Geometry check sheet. Reference: the model listing, model coordinates, mm. A direction names the side the tool comes from. Round coordinates to 2 decimals unless told otherwise and drop trailing zeros. Write each loop counter-clockwise with the first axis right and the second up, starting at its lowest first coordinate (ties: lowest second). Pieces come first, ordered by that corner, then holes. Notation, with made-up numbers: M 37,-39 L 72,-39 A25 cw 72,-18 Z; hole C 3.25,71.25 d9. An arc over 180 degrees is marked long. Answer as CSV lines item,"result". Start each with the question number.
```python
from build123d import *

# Parameters (mm, degrees)
SKETCH1_W                = 150
SKETCH1_H                = 1500
SKETCH1_W_2              = 110
SKETCH1_H_2              = 1460
BOSS_EXTRUDE1_DEPTH      = 20
SKETCH2_W                = 20
SKETCH2_H                = 20
BOSS_EXTRUDE2_DEPTH      = 640
SKETCH3_W                = 150
SKETCH3_H                = 1500
SKETCH3_W_2              = 110
SKETCH3_H_2              = 1460
BOSS_EXTRUDE3_DEPTH      = 20
SKETCH4_W                = 20
SKETCH4_H                = 20
BOSS_EXTRUDE4_DEPTH      = 660
SKETCH5_W                = 20
SKETCH5_H                = 20
BOSS_EXTRUDE5_DEPTH      = 600
BOSS_EXTRUDE5_DEPTH_BACK = 130
SKETCH6_W                = 140
SKETCH6_H                = 20
BOSS_EXTRUDE6_DEPTH      = 20
SKETCH7_W                = 20
SKETCH7_H                = 20
BOSS_EXTRUDE7_DEPTH      = 300
BOSS_EXTRUDE8_START      = -1480
SKETCH8_W                = 20
SKETCH8_H                = 20
BOSS_EXTRUDE8_DEPTH      = 1460


with BuildPart() as part:
    # Sketch1 → Boss-Extrude1 (new body)
    with BuildSketch(Plane(origin=(0, 0, 0), x_dir=(1, 0, 0), z_dir=(0, 1, 0))):
        with Locations((675, 0)):
            Rectangle(SKETCH1_W, SKETCH1_H)
        with Locations((675, 0)):
            Rectangle(SKETCH1_W_2, SKETCH1_H_2, mode=Mode.SUBTRACT)
    extrude(amount=BOSS_EXTRUDE1_DEPTH)

    # Sketch2 → Boss-Extrude2 (add)
    with BuildSketch(Plane(origin=(0, 20, 0), x_dir=(1, 0, 0), z_dir=(0, 1, 0))):
        with Locations((610, 740)):
            Rectangle(SKETCH2_W, SKETCH2_H)
        with Locations((740, 740)):
            Rectangle(SKETCH2_W, SKETCH2_H)
        with Locations((610, -740)):
            Rectangle(SKETCH2_W, SKETCH2_H)
        with Locations((740, -740)):
            Rectangle(SKETCH2_W, SKETCH2_H)
    extrude(amount=BOSS_EXTRUDE2_DEPTH)

    # Sketch3 → Boss-Extrude3 (add)
    with BuildSketch(Plane(origin=(0, 660, 0), x_dir=(1, 0, 0), z_dir=(0, 1, 0))):
        with Locations((675, 0)):
            Rectangle(SKETCH3_W, SKETCH3_H)
        with Locations((675, 0)):
            Rectangle(SKETCH3_W_2, SKETCH3_H_2, mode=Mode.SUBTRACT)
    extrude(amount=BOSS_EXTRUDE3_DEPTH)

    # Sketch4 → Boss-Extrude4 (add)
    with BuildSketch(Plane.XZ):
        with Locations((740, 0)):
            Rectangle(SKETCH4_W, SKETCH4_H)
        with Locations((610, 0)):
            Rectangle(SKETCH4_W, SKETCH4_H)
    extrude(amount=-BOSS_EXTRUDE4_DEPTH)

    # Sketch5 → Boss-Extrude5 (add, two sides)
    with BuildSketch(Plane.ZY.offset(-600)) as boss_extrude5_sk:
        with Locations((-740, 410)):
            Rectangle(SKETCH5_W, SKETCH5_H)
        with Locations((-740, 670)):
            Rectangle(SKETCH5_W, SKETCH5_H)
        with Locations((740, 410)):
            Rectangle(SKETCH5_W, SKETCH5_H)
        with Locations((740, 670)):
            Rectangle(SKETCH5_W, SKETCH5_H)
        with Locations((0, 670)):
            Rectangle(SKETCH5_W, SKETCH5_H)
    extrude(amount=BOSS_EXTRUDE5_DEPTH)
    extrude(boss_extrude5_sk.sketch, amount=-BOSS_EXTRUDE5_DEPTH_BACK)

    # Sketch6 → Boss-Extrude6 (add)
    with BuildSketch(Plane.XZ):
        with Locations((820, 740)):
            Rectangle(SKETCH6_W, SKETCH6_H)
        with Locations((820, 0)):
            Rectangle(SKETCH6_W, SKETCH6_H)
        with Locations((820, -740)):
            Rectangle(SKETCH6_W, SKETCH6_H)
    extrude(amount=-BOSS_EXTRUDE6_DEPTH)

    # Sketch7 → Boss-Extrude7 (add)
    with BuildSketch(Plane.XZ):
        with Locations((610, 740)):
            Rectangle(SKETCH7_W, SKETCH7_H)
        with Locations((880, 740)):
            Rectangle(SKETCH7_W, SKETCH7_H)
        with Locations((610, 0)):
            Rectangle(SKETCH7_W, SKETCH7_H)
        with Locations((610, -740)):
            Rectangle(SKETCH7_W, SKETCH7_H)
        with Locations((880, -740)):
            Rectangle(SKETCH7_W, SKETCH7_H)
        with Locations((880, 0)):
            Rectangle(SKETCH7_W, SKETCH7_H)
    extrude(amount=BOSS_EXTRUDE7_DEPTH)

    # Sketch8 → Boss-Extrude8 (add)
    with BuildSketch(Plane.XY.offset(750).offset(BOSS_EXTRUDE8_START)):
        with Locations((610, -290)):
            Rectangle(SKETCH8_W, SKETCH8_H)
        with Locations((880, -290)):
            Rectangle(SKETCH8_W, SKETCH8_H)
    extrude(amount=BOSS_EXTRUDE8_DEPTH)

    # Mirror1: part across plane


with BuildPart() as part_1:
    add(part.part)
    add(part.part.mirror(Plane(origin=(0, 0, 0), x_dir=(0, 0, 1), z_dir=(1, 0, 0))))


solid = part_1.part
```
1) Section check C-C, the plane z = -349.5. Give the number of separate pieces and of enclosed holes in the cut face, plus the area to 3 significant figures.
2) Go/stop test with flat-tipped pins: pin 1 (16 mm diameter, centred on y = 13.5, z = 478.5, fed in from -X); pin 2 (16 mm diameter, centred on y = 523.5, z = -742, fed in from +X); pin 3 (6 mm diameter, centred on x = 152.5, z = -736.5, fed in from -Y). Record where each tip stops, or that it passes through.
3) Mould release check, pull along Y, two halves, no side actions. Record for faces 1 (the flat face through (4, 410, -730)), 2 (the flat face through (-4, 680, -4)), 3 (the flat face through (872, -86, -730)): released by +Y, released by -Y, zero draft, split by the parting line, or undercut.
4) Scan line: line 1 (Z direction, x = 669, y = 414). Record every from-to range of solid material in increasing order. Write a range as from..to.
5) Section check A-A, the plane x = -193. Record the cut outline in (y, z).
6) Section check B-B, the plane x = -677. Record the cut outline in (y, z).
7) Access from +Z, -Z, +X, -X, +Y, -Y to the whole of each face (thin tool, end or side, straight path). Record for faces 4 (the flat face through (4, 410, 730)), 5 (the flat face through (-750, 495, 4)), 6 (the flat face through (754, 0, 4)).
Results:
1,separate pieces,"12"
1,enclosed holes,"0"
1,area,"4,800 mm^2"
2,pin 1,"stops at x = -750"
2,pin 2,"stops at x = 750"
2,pin 3,"stops at y = 400"
3,face 1,"undercut"
3,face 2,"released by +Y"
3,face 3,"zero draft"
4,line 1,"z = -750..-730, 730..750"
5,outline,"M 400,-750 L 420,-750 L 420,-730 L 400,-730 Z; M 400,730 L 420,730 L 420,750 L 400,750 Z; M 660,-750 L 680,-750 L 680,-730 L 660,-730 Z; M 660,-10 L 680,-10 L 680,10 L 660,10 Z; M 660,730 L 680,730 L 680,750 L 660,750 Z"
6,outline,"M 0,-750 L 20,-750 L 20,-730 L 0,-730 Z; M 0,730 L 20,730 L 20,750 L 0,750 Z; M 400,-750 L 420,-750 L 420,-730 L 400,-730 Z; M 400,730 L 420,730 L 420,750 L 400,750 Z; M 660,-750 L 680,-750 L 680,-730 L 660,-730 Z; M 660,-10 L 680,-10 L 680,10 L 660,10 Z; M 660,730 L 680,730 L 680,750 L 660,750 Z"
7,face 4,"+X, -X"
7,face 5,"+Z, -Z, -X, +Y"
7,face 6,"+Z, -Z, -Y"
